```python
from build123d import *

# Parameters (mm, degrees)
SKETCH1_R                 = 5
EXTRUDE1_DEPTH            = 13.7
M4X0_7_TAPPED_HOLE1_D     = 3.3
M4X0_7_TAPPED_HOLE1_DEPTH = 10
M4X0_7_TAPPED_HOLE1_TIP   = 0.991420021
M4X0_7_TAPPED_HOLE2_D     = 3.3
M4X0_7_TAPPED_HOLE2_DEPTH = 10
M4X0_7_TAPPED_HOLE2_TIP   = 0.991420021
CHAMFER1_SIZE             = 0.25


with BuildPart() as part:
    # Sketch1 → Extrude1 (new body)
    with BuildSketch(Plane.XY):
        Circle(SKETCH1_R)
    extrude(amount=-EXTRUDE1_DEPTH)

    # M4x0.7 Tapped Hole1
    with Locations(Plane.XY):
        with Locations((0, 0)):
            Hole(M4X0_7_TAPPED_HOLE1_D / 2, depth=M4X0_7_TAPPED_HOLE1_DEPTH)
            with Locations((0, 0, -(M4X0_7_TAPPED_HOLE1_DEPTH + M4X0_7_TAPPED_HOLE1_TIP / 2))):  # 118° drill point
                Cone(0, M4X0_7_TAPPED_HOLE1_D / 2, M4X0_7_TAPPED_HOLE1_TIP, mode=Mode.SUBTRACT)

    # M4x0.7 Tapped Hole2
    with Locations(Plane(origin=(0, 0, -13.7), x_dir=(-1, 0, 0), z_dir=(0, 0, -1))):
        with Locations((0, 0)):
            Hole(M4X0_7_TAPPED_HOLE2_D / 2, depth=M4X0_7_TAPPED_HOLE2_DEPTH)
            with Locations((0, 0, -(M4X0_7_TAPPED_HOLE2_DEPTH + M4X0_7_TAPPED_HOLE2_TIP / 2))):  # 118° drill point
                Cone(0, M4X0_7_TAPPED_HOLE2_D / 2, M4X0_7_TAPPED_HOLE2_TIP, mode=Mode.SUBTRACT)

    # Chamfer1
    chamfer1_edges = [part.edges().sort_by_distance(p)[0] for p in [
        (-5, 0, 0),
        (-5, 0, -13.7),
    ]]
    chamfer(chamfer1_edges, length=CHAMFER1_SIZE)


solid = part.part
```
Here's how the part is built. I have some questions about the finished solid (model axes, mm). Coordinates: 2 decimals unless noted, no trailing zeros. Order: outer loops, then holes, each group sorted by start corner. A loop starts at its lowest first (then second) coordinate and runs counter-clockwise, first axis right, second up. Notation, with made-up numbers: (40.25, -11.5) -> (73.25, -11.5) arc R29 cw to (73.25, 27.5) -> close; hole circle Ø2 at (80, 79). An arc over 180 degrees is marked (long way). Return JSON: item names as keys, results as strings.
1) I'm going to push flat-ended pins straight in: P1, Ø2, axis at y = 4, z = -7.5, coming from the -X side; P2, Ø5.5, axis at x = 0, y = 0, coming from the -Z side; P3, Ø2, axis at y = 2, z = -9, coming from the +X side. Where does each tip first touch, or does it pass through?
Conclusion:
{"P1": "stops at x = -4", "P2": "stops at z = -13.7", "P3": "stops at x = 4.9"}
2) If we section it at B-B on z = -1: List the corners of the cut face in (x, y) for me.
Conclusion:
{"outline": "circle Ø10 at (0, 0); hole circle Ø3.3 at (0, 0)"}
3) Thinking about a two-plate mould opening in Z: for faces 1 (the cylindrical face through (-1.08, -4.88, -6.76)), 2 (the flat face through (2, 0, -13.7)), 3 (the flat face through (2, 0, 0)), which applies, +Z half, -Z half, draft (parallel to the pull), parting line (faces both ways), or undercut?
Conclusion:
{"face 1": "draft", "face 2": "-Z half", "face 3": "+Z half"}
4) If I drill on probe 1 along Y at (x, z) = (0, -12.7); probe 2 along Y at (x, z) = (-1.25, -0.75); probe 3 along X at (y, z) = (-1, -9), over which ranges is the centre line in solid material (lowest first)?
Conclusion:
{"probe 1": "y = -5 to -1.65, 1.65 to 5", "probe 2": "y = -4.84 to -1.08, 1.08 to 4.84", "probe 3": "x = -4.9 to -1.31, 1.31 to 4.9"}
5) If we section it at A-A on x = 0: List the corners of the cut face in (y, z) for me.
Conclusion:
{"outline": "(-5, -13.45) -> (-4.75, -13.7) -> (-1.65, -13.7) -> (-1.65, 0) -> (-4.75, 0) -> (-5, -0.25) -> close; (1.65, -13.7) -> (4.75, -13.7) -> (5, -13.45) -> (5, -0.25) -> (4.75, 0) -> (1.65, 0) -> close"}
